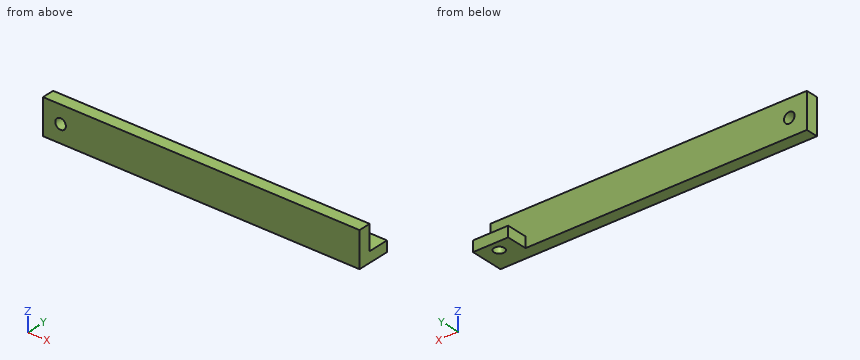
from build123d import *

# Parameters (mm, degrees)
SKETCH1_W           = 90
SKETCH1_H           = 10
SKETCH1_R           = 1.5
BOSS_EXTRUDE1_DEPTH = 3.5
SKETCH2_W           = 10
SKETCH2_H           = 3
BOSS_EXTRUDE2_DEPTH = 6
SKETCH3_R           = 1.5
CUT_EXTRUDE1_DEPTH  = 3


with BuildPart() as part:
    # Sketch1 → Boss-Extrude1 (new body)
    with BuildSketch(Plane(origin=(0, 0, 0), x_dir=(1, 0, 0), z_dir=(0, 1, 0))):
        Rectangle(SKETCH1_W, SKETCH1_H)
        with Locations(Location((-40, 0, 0), (0, 0, 270))):
            Circle(SKETCH1_R, mode=Mode.SUBTRACT)
    extrude(amount=BOSS_EXTRUDE1_DEPTH)

    # Sketch2 → Boss-Extrude2 (add)
    with BuildSketch(Plane(origin=(0, 3.5, 0), x_dir=(1, 0, 0), z_dir=(0, 1, 0))):
        with Locations((40, 3.5)):
            Rectangle(SKETCH2_W, SKETCH2_H)
    extrude(amount=BOSS_EXTRUDE2_DEPTH)

    # Sketch3 → Cut-Extrude1 (cut)
    with BuildSketch(Plane.XY.offset(-2)):
        with Locations((40, 6.5)):
            Circle(SKETCH3_R)
    extrude(amount=-CUT_EXTRUDE1_DEPTH, mode=Mode.SUBTRACT)


solid = part.part
Here's how the part is built. I have some questions about the finished solid (model axes, mm). Give positions to 0.01 mm unless a question says otherwise; leave off trailing zeros. Loops run counter-clockwise (first coordinate to the right, second up) from the corner with the lowest first, then second, coordinate; pieces in that order, holes last. Notation, with made-up numbers: (-29, 43) -> (-24, 43) arc R30 ccw to (-24, 72) -> close; hole circle Ø4 at (-35, -36). An arc over 180 degrees is marked (long way). One line per item, written item: value.
Q1. I'm going to push flat-ended pins straight in: pin 1 Ø0.9 at (y, z) = (6.5, -3) entering from -X; pin 2 Ø3 at (x, z) = (12, 2) entering from +Y. Where does each tip first touch, or does it pass through?
Answers follow:
pin 1: x = 35
pin 2: y = 3.5
Q2. Suppose I cut it at D-D on x = -1.5. Please give me the cut outline in (y, z).
Answers follow:
outline: (0, -5) -> (3.5, -5) -> (3.5, 5) -> (0, 5) -> close
Q3. Suppose I cut it at A-A on x = 40. Please give me the cut outline in (y, z).
Answers follow:
outline: (0, -5) -> (5, -5) -> (5, -2) -> (3.5, -2) -> (3.5, 5) -> (0, 5) -> close; (8, -5) -> (9.5, -5) -> (9.5, -2) -> (8, -2) -> close
Q4. Suppose I cut it at B-B on z = 0. Please give me the cut outline in (x, y), then the cut area to 4 significant figures.
Answers follow:
outline: (-45, 0) -> (-41.5, 0) -> (-41.5, 3.5) -> (-45, 3.5) -> close; (-38.5, 0) -> (45, 0) -> (45, 3.5) -> (-38.5, 3.5) -> close
area: 304.5 mm^2
Q5. If I drill on line 1 along Y through (x, z) = (40, -2.55); line 2 along X through (y, z) = (2.55, 0); line 3 along X through (y, z) = (4, -4.5), over which ranges is the centre line in solid material (lowest first)?
Answers follow:
line 1: 0 to 5, 8 to 9.5
line 2: -45 to -41.5, -38.5 to 45
line 3: 35 to 45
Q6. Suppose I cut it at C-C on x = -40. Please give me the cut outline in (y, z).
Answers follow:
outline: (0, -5) -> (3.5, -5) -> (3.5, -1.5) -> (0, -1.5) -> close; (0, 1.5) -> (3.5, 1.5) -> (3.5, 5) -> (0, 5) -> close
